The listing builds one solid part. Answer for the finished solid, in the listing's coordinates (mm). A direction names the side the tool comes from. Give positions to 0.01 mm unless a question says otherwise; leave off trailing zeros. Loops run counter-clockwise (first coordinate to the right, second up) from the corner with the lowest first, then second, coordinate; pieces in that order, holes last. Notation, with made-up numbers: M 50,69 L 57,69 A24 ccw 57,99 Z; hole C 70,61 d2. An arc over 180 degrees is marked long. One line per item, written item: value. Start each with the question number.
Q1. A cutting plane is placed at C-C, the plane x = 15.5. Determine the outline of the cut face in (y, z).
Q2. For faces 4 (the flat face through (55, -17, 18)), 5 (the flat face through (45, -7.844, 17)), 6 (the flat face through (47.955, -17, 16)), 7 (the flat face through (29, -21, -1)), determine the directions among +Z, -Z, +X, -X, +Y, -Y from which every point of the face is accessible in a straight line to the end or side of a thin tool.
Q3. The mould has two halves that part along Z. Classify faces 1 (the flat face through (30, -16, 18)), 2 (the flat face through (29, -21, 7)), 3 (the flat face through (38.279, -16, 16)): +Z half, -Z half, draft (parallel to the pull), parting line (faces both ways), or undercut.
Q4. A cutting plane is placed at B-B, the plane z = 15.25. Determine the outline of the cut face in (x, y), and give its area (3 significant figures).
Q5. A cutting plane is placed at A-A, the plane y = -11.5. Determine the outline of the cut face in (x, z).
Q6. Consider L1, parallel to X at y = 0, z = 0.25; L2, parallel to Y at x = 58, z = 0.25; L3, parallel to Z at x = 46, y = -16.5. Determine where each line is inside the solid, lowest interval first.
Q7. Flat-ended cylindrical pins translate along their axes: pin 1 (12 mm diameter, centred on x = 42, y = -7, fed in from -Z); pin 2 (2 mm diameter, centred on y = -16.5, z = 16, fed in from -X); pin 3 (9.5 mm diameter, centred on x = 24.5, y = -12, fed in from +Z). Find the tip coordinate at first contact, or state that the pin passes through.
Q8. A cutting plane is placed at D-D, the plane y = -6. Determine the outline of the cut face in (x, z), and give its area (3 significant figures).
Autodesk Inventor part; units mm, degrees
ref_plane "YZ Plane" through (0, 0, 0) normal (1, 0, 0) x (0, 1, 0)
ref_plane "XZ Plane" through (0, 0, 0) normal (0, 1, 0) x (-1, 0, 0)
ref_plane "XY Plane" through (0, 0, 0) normal (0, 0, 1) x (1, 0, 0)
sketch "스케치1" plane through (0, 0, 0) normal (0, 0, 1) x (1, 0, 0)
  circle A0 centre (0, 0) radius 1.4
  line L0 (0, 0) -> (58, 0)
  line L1 (58, 0) -> (58, -23)
  circle A1 centre (58, 0) radius 1.4
  circle A2 centre (0, -23) radius 1.4
  circle A3 centre (58, -23) radius 1.4
  line L2 (0, 0) -> (0, 4)
  line L3 (0, 4) -> (-4, 4)
  line L4 (0, 4) -> (58, 4)
  line L5 (62, 0) -> (62, -23)
  line L6 (58, -27) -> (0, -27)
  line L7 (-4, -23) -> (-4, 0)
  arc A4 (0, 4) -> (-4, 0) centre (0, 0) ccw
  arc A5 (62, 0) -> (58, 4) centre (58, 0) ccw
  arc A6 (58, -27) -> (62, -23) centre (58, -23) ccw
  arc A7 (-4, -23) -> (0, -27) centre (0, -23) ccw
  point P0 (62, -27)
  point P1 (62, 4)
  point P2 (-4, -27)
  dimension "d0" = 2.8
  dimension "d1" = 58
  dimension "d2" = 23
  dimension "d5" = 58
  dimension "d8" = 23
  dimension "d11" = 4
  dimension "d12" = 4
  dimension "d13" = 66
  dimension "d14" = 31
  dimension "d21" = 4
extrude "돌출1" add sketch "스케치1" along normal blind 14
extrude "돌출2" cut sketch "스케치1" along normal blind 13
extrude "돌출3" add sketch "스케치1" along normal blind 1.5
sketch "스케치2" plane through (0, 0, 14) normal (0, 0, 1) x (1, 0, 0)
  line L0 (58, 4) -> (0, 4)
  line L1 (39.5003, 4) -> (50.7727, 4)
  line L2 (50.7727, 4) -> (50.7727, -7.8437)
  line L3 (50.7727, -7.8437) -> (39.5003, -7.8437)
  line L4 (39.5003, -7.8437) -> (39.5003, 4)
  line L5 (62, -23) -> (62, 0)
  line L6 (62, -4.9317) -> (50.7727, -4.9317)
  line L7 (50.7727, -4.9317) -> (50.7727, -14.5132)
  line L8 (50.7727, -14.5132) -> (62, -14.5132)
  line L9 (62, -14.5132) -> (62, -4.9317)
  line L10 (62, -14.5132) -> (47.9546, -14.5132)
  line L11 (47.9546, -14.5132) -> (47.9546, -19.3979)
  line L12 (47.9546, -19.3979) -> (62, -19.3979)
  line L13 (62, -19.3979) -> (62, -14.5132)
  line L14 (38.2792, -12.8223) -> (25.0341, -12.8223)
  line L15 (25.0341, -12.8223) -> (25.0341, -18.4585)
  line L16 (25.0341, -18.4585) -> (38.2792, -18.4585)
  line L17 (38.2792, -18.4585) -> (38.2792, -12.8223)
  point P0 (0, 0)
  point P1 (50.7727, -7.8437)
extrude "돌출4" add sketch "스케치2" along normal blind 6 contours L2 L3 L4 L0 | L6 L5 L8 L7 L2
extrude "돌출5" add sketch "스케치2" along normal blind 4 contours L8 L5 L12 L11 L10 | L17 L16 L15 L14
sketch "스케치3" plane through (0, 0, 1.5) normal (0, 0, 1) x (1, 0, 0)
  line L0 (0, -27) -> (58, -27)
  line L1 (29, -27) -> (4, -27)
  line L2 (4, -27) -> (54, -27)
  line L3 (54, -27) -> (54, -21)
  line L4 (54, -21) -> (4, -21)
  line L5 (4, -21) -> (4, -27)
  point P0 (0, 0)
  dimension "d26" = 25
  dimension "d27" = 50
  dimension "d28" = 6
extrude "돌출6" add sketch "스케치3" along normal blind 12.25
extrude "돌출7" add sketch "스케치1" along normal blind 9.5
sketch "스케치4" plane through (0, 0, 0) normal (0, 0, -1) x (-1, 0, 0)
  line L0 (-4, -21) -> (-4, -27)
  line L1 (-4, -21) -> (-4, -27)
  line L2 (-54, -27) -> (-54, -21)
  line L3 (-54, -27) -> (-54, -21)
  line L4 (-54, -21) -> (-4, -21)
  line L5 (-54, -21) -> (-4, -21)
  line L6 (-4, -21) -> (-4, -27)
  line L7 (-4, -27) -> (-54, -27)
  line L8 (-54, -27) -> (-54, -21)
  point P0 (0, 0)
extrude "돌출8" add sketch "스케치4" along normal blind 2
sketch "스케치5" plane through (0, 0, 14) normal (0, 0, 1) x (1, 0, 0)
  circle A0 centre (0, 0) radius 2.2
  line L0 (2.2, 0) -> (2.2, 3)
  line L1 (58, 4) -> (0, 4)
  line L2 (2.2, 3) -> (24.2, 3)
  line L3 (24.2, 3) -> (24.2, -4.2)
  line L4 (24.2, -4.2) -> (2.2, -4.2)
  line L5 (2.2, -4.2) -> (2.2, 3)
  dimension "d35" = 4.4
  dimension "d36" = 3
  dimension "d37" = 22
  dimension "d38" = 7.2
extrude "돌출9" add sketch "스케치5" along normal blind 2.5 contours L0 L2 L3 L4 L5
move faces "이동1" translate (-4, 0, 0) faces at (25.0341, -14.7011, 15.3333)
move faces "이동2" translate (0, 0, -9) faces at (37.3333, -7.2234, 9.5)
properties part number "라파+hat"
Answer block:
1. outline: M -27,-2 L -21,-2 L -21,0 L 4,0 L 4,0.5 L -21,0.5 L -21,13 L 4,13 L 4,14 L 3,14 L 3,16.5 L -4.2,16.5 L -4.2,14 L -27,14 Z
2. face 4: +Z, +X, -X, -Y
2. face 5: +Z, -X
2. face 6: +Z, -Y
2. face 7: -Z, +X, -X, +Y
3. face 1: +Z half
3. face 2: undercut
3. face 3: draft
4. outline: M 2.2,-4.2 L 24.2,-4.2 L 24.2,3 L 2.2,3 Z; M 21.03,-18.46 L 38.28,-18.46 L 38.28,-12.82 L 21.03,-12.82 Z; M 39.5,-7.84 L 50.77,-7.84 L 50.77,-14.51 L 47.95,-14.51 L 47.95,-19.4 L 62,-19.4 L 62,-4.93 L 50.77,-4.93 L 50.77,4 L 39.5,4 Z
4. area: 565 mm^2
5. outline: M -4,0 L 62,0 L 62,0.5 L -4,0.5 Z; M -4,13 L 62,13 L 62,20 L 50.77,20 L 50.77,14 L -4,14 Z
6. L1: -4 to -1.4, 1.4 to 56.6, 59.4 to 62
6. L2: -27 to -24.4, -21.6 to -1.4, 1.4 to 4
6. L3: 0 to 0.5, 13 to 14
7. pin 1: z = 0
7. pin 2: x = 21.03
7. pin 3: z = 18
8. outline: M -4,0 L 62,0 L 62,0.5 L -4,0.5 Z; M -4,13 L 62,13 L 62,20 L 39.5,20 L 39.5,14 L -4,14 Z
8. area: 234 mm^2
